Source: CAD feature listing. Evaluate the final solid. Frame: model axes, mm. Face numbers are marked on the shaded views. A direction names the side the tool comes from. Round coordinates to 2 decimals unless told otherwise and drop trailing zeros. Write each loop counter-clockwise with the first axis right and the second up, starting at its lowest first coordinate (ties: lowest second). Pieces come first, ordered by that corner, then holes.
from build123d import *

# Parameters (mm, degrees)
SKETCH1_W           = 51
SKETCH1_H           = 22
SKETCH1_R           = 1.25
BOSS_EXTRUDE1_DEPTH = 1.8
SKETCH2_R           = 8
BOSS_EXTRUDE2_DEPTH = 13


with BuildPart() as part:
    # Sketch1 → Boss-Extrude1 (new body)
    with BuildSketch(Plane.XY):
        Rectangle(SKETCH1_W, SKETCH1_H)
        with Locations((-23, -8.5)):
            Circle(SKETCH1_R, mode=Mode.SUBTRACT)
        with Locations((-23, 8.5)):
            Circle(SKETCH1_R, mode=Mode.SUBTRACT)
        with Locations((23, 8.5)):
            Circle(SKETCH1_R, mode=Mode.SUBTRACT)
        with Locations((23, -8.5)):
            Circle(SKETCH1_R, mode=Mode.SUBTRACT)
    extrude(amount=BOSS_EXTRUDE1_DEPTH)

    # Sketch2 → Boss-Extrude2 (add)
    with BuildSketch(Plane.XY.offset(1.8)):
        with Locations((-17, 0)):
            Circle(SKETCH2_R)
        with Locations((17, 0)):
            Circle(SKETCH2_R)
    extrude(amount=BOSS_EXTRUDE2_DEPTH)


solid = part.part
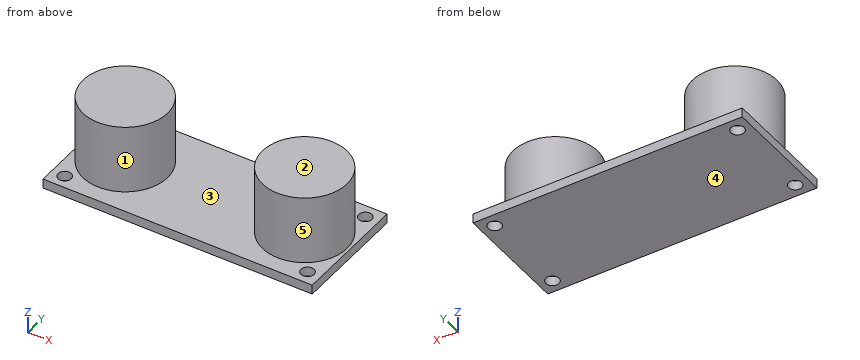
1) Section query C-C on y = 0. Return the cut outline in (x, z), then the cut area to 3 significant figures.
Taken from the geometry:
outline: (-25.5, 0) - (25.5, 0) - (25.5, 1.8) - (25, 1.8) - (25, 14.8) - (9, 14.8) - (9, 1.8) - (-9, 1.8) - (-9, 14.8) - (-25, 14.8) - (-25, 1.8) - (-25.5, 1.8) - close
area: 508 mm2
2) Section query A-A on y = 8.5. Return the cut outline in (x, z), then the cut area to 3 significant figures.
Taken from the geometry:
outline: (-25.5, 0) - (-24.25, 0) - (-24.25, 1.8) - (-25.5, 1.8) - close; (-21.75, 0) - (21.75, 0) - (21.75, 1.8) - (-21.75, 1.8) - close; (24.25, 0) - (25.5, 0) - (25.5, 1.8) - (24.25, 1.8) - close
area: 82.8 mm2
3) Contact query for flat-ended pins moving along their axis: P1, Ø5, axis at y = 6.5, z = 9, coming from the -X side; P2, Ø1, axis at x = -15.5, z = 6, coming from the -Y side. Output: stop coordinate, or through.
Taken from the geometry:
P1: stops at x = -23.93
P2: stops at y = -7.94
4) Reachability of the marked faces 1 and 2 from +Z, -Z, +X, -X, +Y, -Y: full face, straight path, thin tool, end or side. Return the list, or none.
Taken from the geometry:
face 1: +Z
face 2: +Z, +X, -X, +Y, -Y
5) Section query D-D on z = 4.5. Return the cut outline in (x, y).
Taken from the geometry:
outline: circle Ø16 at (-17, 0); circle Ø16 at (17, 0)
6) Section query B-B on x = -17. Return the cut outline in (y, z), then the cut area to 3 significant figures.
Taken from the geometry:
outline: (-11, 0) - (11, 0) - (11, 1.8) - (8, 1.8) - (8, 14.8) - (-8, 14.8) - (-8, 1.8) - (-11, 1.8) - close
area: 248 mm2
7) Pull-direction query (X, two-part tool) for the marked faces 3, 4 and 5; classes: released by +X, released by -X, zero draft, split by the parting line, or undercut.
Taken from the geometry:
face 3: undercut
face 4: zero draft
face 5: undercut
8) Material intervals for line 1 (Y direction, x = 23, z = 0.6); line 2 (Z direction, x = -3, y = -6.75); line 3 (X direction, y = -2, z = 6.75), sorted ascending.
Taken from the geometry:
line 1: y = -11 to -9.75, -7.25 to 7.25, 9.75 to 11
line 2: z = 0 to 1.8
line 3: x = -24.75 to -9.25, 9.25 to 24.75
